```python
from build123d import *

# Parameters (mm, degrees)
SKETCH1_W           = 300
SKETCH1_H           = 150
BOSS_EXTRUDE1_DEPTH = 125
SKETCH2_W           = 270
SKETCH2_H           = 120
CUT_EXTRUDE1_DEPTH  = 110
SKETCH4_R           = 2.5
CUT_EXTRUDE5_DEPTH  = 350
SKETCH6_R           = 2.5
CUT_EXTRUDE6_DEPTH  = 175
FILLET1_R           = 5
FILLET2_R           = 5
FILLET3_R           = 5
FILLET4_R           = 5
FILLET5_R           = 2
SKETCH7_R           = 37.5
CUT_EXTRUDE7_DEPTH  = 25
SKETCH8_R           = 45
CUT_EXTRUDE8_DEPTH  = 5
SKETCH9_R           = 37.5
CUT_EXTRUDE9_DEPTH  = 20
BOSS_EXTRUDE2_DEPTH = 5
SKETCH12_R          = 2.0701
CUT_EXTRUDE10_DEPTH = 12.7


with BuildPart() as part:
    # Sketch1 → Boss-Extrude1 (new body)
    with BuildSketch(Plane(origin=(0, 0, 0), x_dir=(1, 0, 0), z_dir=(0, 1, 0))):
        Rectangle(SKETCH1_W, SKETCH1_H)
    extrude(amount=BOSS_EXTRUDE1_DEPTH)

    # Sketch2 → Cut-Extrude1 (cut)
    with BuildSketch(Plane.XZ):
        Rectangle(SKETCH2_W, SKETCH2_H)
    extrude(amount=-CUT_EXTRUDE1_DEPTH, mode=Mode.SUBTRACT)

    # Sketch4 → Cut-Extrude5 (cut)
    with BuildSketch(Plane(origin=(150, 0, 0), x_dir=(0, 0, -1), z_dir=(1, 0, 0))):
        with Locations((-52.5, 7.5)):
            Circle(SKETCH4_R)
        with Locations((52.5, 7.5)):
            Circle(SKETCH4_R)
    extrude(amount=-CUT_EXTRUDE5_DEPTH, mode=Mode.SUBTRACT)

    # Sketch6 → Cut-Extrude6 (cut)
    with BuildSketch(Plane.XY.offset(75)):
        with Locations((-130, 105)):
            Circle(SKETCH6_R)
        with Locations((130, 105)):
            Circle(SKETCH6_R)
    extrude(amount=-CUT_EXTRUDE6_DEPTH, mode=Mode.SUBTRACT)

    # Fillet1
    # the kernel refuses this fillet: 5 mm, written as the material it adds along each edge
    with BuildSketch(Plane(origin=(147.5, 110, -60), x_dir=(0, -1, 0), z_dir=(-1, 0, 0))) as fillet1_piece_1_section:
        with BuildLine():
            CenterArc((FILLET1_R, FILLET1_R), FILLET1_R, 180, 90)
            Line((0, FILLET1_R), (0, 0))
            Line((0, 0), (FILLET1_R, 0))
        make_face()
    fillet1_piece_1 = extrude(amount=295, mode=Mode.PRIVATE)
    fillet1_piece_1 = fillet1_piece_1 - Plane(origin=(130, 105, -58.868024429), x_dir=(1, 0, 0), z_dir=(0, 0, 1)) * Cylinder(2.5, 610, mode=Mode.PRIVATE)
    fillet1_piece_1 = fillet1_piece_1 - Plane(origin=(-130, 105, -58.868024429), x_dir=(1, 0, 0), z_dir=(0, 0, 1)) * Cylinder(2.5, 610, mode=Mode.PRIVATE)
    add(fillet1_piece_1)

    # Fillet2
    # the kernel refuses this fillet: 5 mm, written as the material it adds along each edge
    with BuildSketch(Plane(origin=(-147.5, 110, 60), x_dir=(0, 0, -1), z_dir=(1, 0, 0))) as fillet2_piece_1_section:
        with BuildLine():
            CenterArc((FILLET2_R, -FILLET2_R), FILLET2_R, 90, 90)
            Line((0, -FILLET2_R), (0, 0))
            Line((0, 0), (FILLET2_R, 0))
        make_face()
    fillet2_piece_1 = extrude(amount=295, mode=Mode.PRIVATE)
    fillet2_piece_1 = fillet2_piece_1 - Plane(origin=(-130, 105, 58.868024429), x_dir=(1, 0, 0), z_dir=(0, 0, 1)) * Cylinder(2.5, 610, mode=Mode.PRIVATE)
    fillet2_piece_1 = fillet2_piece_1 - Plane(origin=(130, 105, 58.868024429), x_dir=(1, 0, 0), z_dir=(0, 0, 1)) * Cylinder(2.5, 610, mode=Mode.PRIVATE)
    add(fillet2_piece_1)

    # Fillet3
    # the kernel refuses this fillet: 5 mm, written as the material it adds along each edge
    with BuildSketch(Plane(origin=(-135, 0, 60), x_dir=(0, 0, -1), z_dir=(0, 1, 0))) as fillet3_piece_1_section:
        with BuildLine():
            CenterArc((FILLET3_R, -FILLET3_R), FILLET3_R, 90, 90)
            Line((0, -FILLET3_R), (0, 0))
            Line((0, 0), (FILLET3_R, 0))
        make_face()
    fillet3_piece_1 = extrude(amount=105, mode=Mode.PRIVATE)
    fillet3_piece_1 = fillet3_piece_1 - Plane(origin=(-130, 105, 58.86600748), x_dir=(1, 0, 0), z_dir=(0, 0, 1)) * Cylinder(2.5, 230, mode=Mode.PRIVATE)
    add(fillet3_piece_1)
    with BuildSketch(Plane(origin=(-135, 105, 55), x_dir=(0, 0, 1), z_dir=(0, -1, 0))) as fillet3_piece_2_section:
        with BuildLine():
            CenterArc((5 - FILLET3_R, -FILLET3_R), FILLET3_R, 0, 90)
            Line((5 - FILLET3_R, 0), (5, 0))
            Line((5, 0), (5, -FILLET3_R))
        make_face()
    fillet3_piece_2 = revolve(axis=Axis((-135, 105, 55), (-1, 0, 0)), revolution_arc=90, mode=Mode.PRIVATE)
    fillet3_piece_2 = fillet3_piece_2 - Plane(origin=(-130, 105, 57.577819165), x_dir=(1, 0, 0), z_dir=(0, 0, 1)) * Cylinder(2.5, 20, mode=Mode.PRIVATE)
    add(fillet3_piece_2)
    with BuildSketch(Plane(origin=(-135, 0, -60), x_dir=(0, 0, 1), z_dir=(0, 1, 0))) as fillet3_piece_3_section:
        with BuildLine():
            CenterArc((FILLET3_R, FILLET3_R), FILLET3_R, 180, 90)
            Line((0, FILLET3_R), (0, 0))
            Line((0, 0), (FILLET3_R, 0))
        make_face()
    fillet3_piece_3 = extrude(amount=105, mode=Mode.PRIVATE)
    fillet3_piece_3 = fillet3_piece_3 - Plane(origin=(-130, 105, -58.86600748), x_dir=(1, 0, 0), z_dir=(0, 0, 1)) * Cylinder(2.5, 231, mode=Mode.PRIVATE)
    add(fillet3_piece_3)
    with BuildSketch(Plane(origin=(-135, 105, -55), x_dir=(0, 0, -1), z_dir=(0, -1, 0))) as fillet3_piece_4_section:
        with BuildLine():
            CenterArc((5 - FILLET3_R, FILLET3_R), FILLET3_R, 270, 90)
            Line((5, FILLET3_R), (5, 0))
            Line((5, 0), (5 - FILLET3_R, 0))
        make_face()
    fillet3_piece_4 = revolve(axis=Axis((-135, 105, -55), (1, 0, 0)), revolution_arc=90, mode=Mode.PRIVATE)
    fillet3_piece_4 = fillet3_piece_4 - Plane(origin=(-130, 105, -57.577819165), x_dir=(1, 0, 0), z_dir=(0, 0, 1)) * Cylinder(2.5, 20, mode=Mode.PRIVATE)
    add(fillet3_piece_4)
    with BuildSketch(Plane(origin=(-135, 110, -55), x_dir=(0, -1, 0), z_dir=(0, 0, 1))) as fillet3_piece_5:
        with BuildLine():
            CenterArc((FILLET3_R, FILLET3_R), FILLET3_R, 180, 90)
            Line((0, FILLET3_R), (0, 0))
            Line((0, 0), (FILLET3_R, 0))
        make_face()
    extrude(amount=110)

    # Fillet4
    # the kernel refuses this fillet: 5 mm, written as the material it adds along each edge
    with BuildSketch(Plane(origin=(135, 0, -60), x_dir=(0, 0, 1), z_dir=(0, 1, 0))) as fillet4_piece_1_section:
        with BuildLine():
            CenterArc((FILLET4_R, -FILLET4_R), FILLET4_R, 90, 90)
            Line((0, -FILLET4_R), (0, 0))
            Line((0, 0), (FILLET4_R, 0))
        make_face()
    fillet4_piece_1 = extrude(amount=105, mode=Mode.PRIVATE)
    fillet4_piece_1 = fillet4_piece_1 - Plane(origin=(130, 105, -58.866007422), x_dir=(1, 0, 0), z_dir=(0, 0, 1)) * Cylinder(2.5, 231, mode=Mode.PRIVATE)
    add(fillet4_piece_1)
    with BuildSketch(Plane(origin=(135, 105, -55), x_dir=(0, 0, -1), z_dir=(0, -1, 0))) as fillet4_piece_2_section:
        with BuildLine():
            CenterArc((5 - FILLET4_R, -FILLET4_R), FILLET4_R, 0, 90)
            Line((5 - FILLET4_R, 0), (5, 0))
            Line((5, 0), (5, -FILLET4_R))
        make_face()
    fillet4_piece_2 = revolve(axis=Axis((135, 105, -55), (1, 0, 0)), revolution_arc=90, mode=Mode.PRIVATE)
    fillet4_piece_2 = fillet4_piece_2 - Plane(origin=(130, 105, -57.577819011), x_dir=(1, 0, 0), z_dir=(0, 0, 1)) * Cylinder(2.5, 20, mode=Mode.PRIVATE)
    add(fillet4_piece_2)
    with BuildSketch(Plane(origin=(135, 0, 60), x_dir=(0, 0, -1), z_dir=(0, 1, 0))) as fillet4_piece_3_section:
        with BuildLine():
            CenterArc((FILLET4_R, FILLET4_R), FILLET4_R, 180, 90)
            Line((0, FILLET4_R), (0, 0))
            Line((0, 0), (FILLET4_R, 0))
        make_face()
    fillet4_piece_3 = extrude(amount=105, mode=Mode.PRIVATE)
    fillet4_piece_3 = fillet4_piece_3 - Plane(origin=(130, 105, 58.866007422), x_dir=(1, 0, 0), z_dir=(0, 0, 1)) * Cylinder(2.5, 231, mode=Mode.PRIVATE)
    add(fillet4_piece_3)
    with BuildSketch(Plane(origin=(135, 105, 55), x_dir=(0, 0, 1), z_dir=(0, -1, 0))) as fillet4_piece_4_section:
        with BuildLine():
            CenterArc((5 - FILLET4_R, FILLET4_R), FILLET4_R, 270, 90)
            Line((5, FILLET4_R), (5, 0))
            Line((5, 0), (5 - FILLET4_R, 0))
        make_face()
    fillet4_piece_4 = revolve(axis=Axis((135, 105, 55), (-1, 0, 0)), revolution_arc=90, mode=Mode.PRIVATE)
    fillet4_piece_4 = fillet4_piece_4 - Plane(origin=(130, 105, 57.577819011), x_dir=(1, 0, 0), z_dir=(0, 0, 1)) * Cylinder(2.5, 20, mode=Mode.PRIVATE)
    add(fillet4_piece_4)
    with BuildSketch(Plane(origin=(135, 110, 55), x_dir=(-1, 0, 0), z_dir=(0, 0, -1))) as fillet4_piece_5:
        with BuildLine():
            CenterArc((FILLET4_R, -FILLET4_R), FILLET4_R, 90, 90)
            Line((0, -FILLET4_R), (0, 0))
            Line((0, 0), (FILLET4_R, 0))
        make_face()
    extrude(amount=110)

    # Fillet5
    fillet5_edges = [part.edges().sort_by_distance(p)[0] for p in [
        (-133.535533906, 0, 58.535533906),
        (-133.535533906, 0, -58.535533906),
        (135, 0, 0),
        (0, 0, 60),
        (133.535533906, 0, -58.535533906),
        (133.535533906, 0, 58.535533906),
        (-135, 0, 0),
        (0, 0, -60),
    ]]
    fillet(fillet5_edges, radius=FILLET5_R)

    # Sketch7 → Cut-Extrude7 (cut)
    with BuildSketch(Plane(origin=(150, 0, 0), x_dir=(0, 0, -1), z_dir=(1, 0, 0))):
        with Locations((0, 55)):
            Circle(SKETCH7_R)
    extrude(amount=-CUT_EXTRUDE7_DEPTH, mode=Mode.SUBTRACT)

    # Sketch8 → Cut-Extrude8 (cut)
    with BuildSketch(Plane.ZY.offset(-135)):
        with Locations((0, 55)):
            Circle(SKETCH8_R)
    extrude(amount=-CUT_EXTRUDE8_DEPTH, mode=Mode.SUBTRACT)

    # Sketch9 → Cut-Extrude9 (cut)
    with BuildSketch(Plane(origin=(150, 0, 0), x_dir=(0, 0, -1), z_dir=(1, 0, 0))):
        with Locations((0, 55)):
            Circle(SKETCH9_R)
        with BuildLine():
            Line((0, 55), (-43.817091414, 65.25))
            ThreePointArc((-43.817091414, 65.25), (-45, 55), (-43.817091414, 44.75))
            Line((-43.817091414, 44.75), (0, 55))
        make_face()
        with BuildLine():
            ThreePointArc((43.817091414, 65.25), (45, 55), (43.817091414, 44.75))
            Line((43.817091414, 44.75), (0, 55))
            Line((0, 55), (43.817091414, 65.25))
        make_face()
    extrude(amount=-CUT_EXTRUDE9_DEPTH, mode=Mode.SUBTRACT)

    # Sketch10 → Boss-Extrude2 (add)
    with BuildSketch(Plane.ZY.offset(-140)):
        with BuildLine():
            Line((-3.5, 99.863682417), (-3.5, 92.336309405))
            ThreePointArc((-3.5, 92.336309405), (0, 92.5), (3.5, 92.336309405))
            Line((3.5, 92.336309405), (3.5, 99.863682417))
            ThreePointArc((3.5, 99.863682417), (0, 100), (-3.5, 99.863682417))
        make_face()
    extrude(amount=BOSS_EXTRUDE2_DEPTH)

    # Sketch12 → Cut-Extrude10 (cut)
    with BuildSketch(Plane.XZ):
        with Locations(Location((144.7549, 69.7549, 0), (0, 0, 270))):
            Circle(SKETCH12_R)
        with Locations(Location((144.7549, -69.7549, 0), (0, 0, 90))):
            Circle(SKETCH12_R)
        with Locations(Location((-144.7549, -69.7549, 0), (0, 0, 270))):
            Circle(SKETCH12_R)
        with Locations(Location((-144.7549, 69.7549, 0), (0, 0, 90))):
            Circle(SKETCH12_R)
    extrude(amount=-CUT_EXTRUDE10_DEPTH, mode=Mode.SUBTRACT)


solid = part.part
```
Can you work these out from the model? Positions are in its coordinate system, mm. A direction names the side the tool comes from. Coordinates: 2 decimals unless noted, no trailing zeros. Loops run counter-clockwise (first coordinate to the right, second up) from the corner with the lowest first, then second, coordinate; pieces in that order, holes last.
1) Imagine slicing it at A-A on z = 0. List the corners of the cut face in (x, y) for me, plus the area to 3 significant figures.
2) Imagine slicing it at B-B on x = 9. List the corners of the cut face in (y, z) for me.
3) Imagine slicing it at C-C on y = 55. List the corners of the cut face in (x, z) for me.
4) I need wall thicknesses on probe 1 along X at (y, z) = (105, 68); probe 2 along Z at (x, y) = (-19, 29); probe 3 along X at (y, z) = (13, 4). Which ranges of each line are inside material? Lowest first, please.
5) Imagine slicing it at D-D on z = -22.5. List the corners of the cut face in (x, y) for me.
6) Which directions (+Z, -Z, +X, -X, +Y, -Y) give clear straight access to the entire face, cutting with the end or side of a thin tool? Please do faces 5 (the flat face through (145.07, 45.59, -40.22)), 6 (the flat face through (-2, 62, 75)), 7 (the flat face through (-2, 53, 60)), 8 (the flat face through (140, 17.5, -3.5)).
7) For pin 1 (4 mm diameter, centred on y = 7.5, z = 52.5, fed in from +X); pin 2 (3.5 mm diameter, centred on x = 144.75, z = 69.75, fed in from -Y); pin 3 (3 mm diameter, centred on x = 24.5, z = 36, fed in from -Y); pin 4 (1 mm diameter, centred on y = 63, z = -12, fed in from +X), each with a flat end and sliding along its axis, tell me the tip position at first contact or that it passes through.
8) Thinking about a two-plate mould opening in Y: for faces 1 (the flat face through (140, 83.1, -25.2)), 2 (the flat face through (135, 7, -1)), 3 (the flat face through (-1, 0, -67)), 4 (the cylindrical face through (139.06, 47.55, -44.38)), which applies, pulls with the +Y half, pulls with the -Y half, needs draft (parallel to the pull), parting line crosses it, or undercut?
Completed:
1. outline: (-150, 0) - (-137, 0) arc R2 ccw to (-135, 2) - (-135, 105) arc R5 cw to (-130, 110) - (130, 110) arc R5 cw to (135, 105) - (135, 92.5) - (150, 92.5) - (150, 125) - (-150, 125) - close; (135, 2) arc R2 ccw to (137, 0) - (150, 0) - (150, 17.5) - (140, 17.5) - (140, 10) - (135, 10) - close
1. area: 6,650 mm2
2. outline: (0, -75) - (125, -75) - (125, 75) - (0, 75) - (0, 62) arc R2 ccw to (2, 60) - (105, 60) arc R5 cw to (110, 55) - (110, -55) arc R5 cw to (105, -60) - (2, -60) arc R2 ccw to (0, -62) - close
3. outline: (-150, -75) - (150, -75) - (150, -45) - (135, -45) - (135, -55) arc R5 cw to (130, -60) - (-130, -60) arc R5 cw to (-135, -55) - (-135, 55) arc R5 cw to (-130, 60) - (130, 60) arc R5 cw to (135, 55) - (135, 45) - (150, 45) - (150, 75) - (-150, 75) - close
4. probe 1: x = -150 to -132.5, -127.5 to 127.5, 132.5 to 150
4. probe 2: z = -75 to -60, 60 to 75
4. probe 3: x = -150 to -135, 140 to 150
5. outline: (-150, 0) - (-137, 0) arc R2 ccw to (-135, 2) - (-135, 105) arc R5 cw to (-130, 110) - (130, 110) arc R5 cw to (135, 105) - (135, 93.97) - (140, 93.97) - (140, 85) - (150, 85) - (150, 125) - (-150, 125) - close; (135, 2) arc R2 ccw to (137, 0) - (150, 0) - (150, 25) - (140, 25) - (140, 16.03) - (135, 16.03) - close
6. face 5: +X
6. face 6: +Z, +X, -X, +Y, -Y
6. face 7: -Y
6. face 8: none
7. pin 1: passes through
7. pin 2: stops at y = 12.7
7. pin 3: stops at y = 110
7. pin 4: stops at x = -135
8. face 1: undercut
8. face 2: needs draft
8. face 3: pulls with the -Y half
8. face 4: undercut
